Part model, mm, in its own coordinate system. A direction names the side the tool comes from. Round coordinates to 2 decimals unless told otherwise and drop trailing zeros.
(1) Cut at A-A on y = -2.5. Count the separate pieces of the cut face and the enclosed holes in it, then the cut area to 3 significant figures.
(2) Tool access for faces 1 (the face through (2, -6.5, 2)), 2 (the face through (-17, -3.5, 1)): list every direction of +Z, -Z, +X, -X, +Y, -Y with a clear straight run to the whole face (end or side of a thin tool).
(3) Mould opens along Z. For faces 3 (the face through (-77, -3.5, 1)), 4 (the face through (2, -3, -4.5)), 5 (the face through (-150, -3, 0)) say: +Z half, -Z half, draft (parallel to the pull), parting line (faces both ways), or undercut.
(4) Flat gauge pins, fed straight in: pin 1 (3 mm diameter, centred on x = -120, z = -0.5, fed in from +Y); pin 2 (1.8 mm diameter, centred on x = 81.5, z = 0, fed in from -Y); pin 3 (3.5 mm diameter, centred on x = -138.5, z = 0, fed in from +Y). Where does each tip first touch, or does it go through?
(5) Probe probe 1 along Z at (x, y) = (141.5, -2.3); probe 2 along Z at (x, y) = (-78.5, -4.7); probe 3 along Y at (x, z) = (120, -2). List the from-to ranges inside material, lowest first.
from build123d import *

# Parameters (mm, degrees)
SKETCH1_W           = 9
SKETCH1_H           = 6.5
BOSS_EXTRUDE1_DEPTH = 150
SKETCH2_R           = 1.5
CUT_EXTRUDE1_DEPTH  = 151.208188858
SKETCH3_R           = 3
CUT_EXTRUDE2_DEPTH  = 3.5


with BuildPart() as part:
    # Sketch1 → Boss-Extrude1 (new, symmetric)
    with BuildSketch(Plane(origin=(0, 0, 0), x_dir=(0, 0, -1), z_dir=(1, 0, 0))):
        with Locations((0, -3.25)):
            Rectangle(SKETCH1_W, SKETCH1_H)
    extrude(amount=BOSS_EXTRUDE1_DEPTH, both=True)

    # Sketch2 → Cut-Extrude1 (cut, through all)
    with BuildSketch(Plane(origin=(0, 0, 0), x_dir=(1, 0, 0), z_dir=(0, 1, 0))):
        with Locations(Location((-138.5, 0, 0), (0, 0, 270))):
            Circle(SKETCH2_R)
        with Locations(Location((-118.5, 0, 0), (0, 0, 270))):
            Circle(SKETCH2_R)
        with Locations(Location((-98.5, 0, 0), (0, 0, 270))):
            Circle(SKETCH2_R)
        with Locations(Location((-78.5, 0, 0), (0, 0, 270))):
            Circle(SKETCH2_R)
        with Locations(Location((-58.5, 0, 0), (0, 0, 270))):
            Circle(SKETCH2_R)
        with Locations(Location((-38.5, 0, 0), (0, 0, 270))):
            Circle(SKETCH2_R)
        with Locations(Location((-18.5, 0, 0), (0, 0, 270))):
            Circle(SKETCH2_R)
        with Locations(Location((1.5, 0, 0), (0, 0, 270))):
            Circle(SKETCH2_R)
        with Locations(Location((21.5, 0, 0), (0, 0, 270))):
            Circle(SKETCH2_R)
        with Locations(Location((41.5, 0, 0), (0, 0, 270))):
            Circle(SKETCH2_R)
        with Locations(Location((61.5, 0, 0), (0, 0, 270))):
            Circle(SKETCH2_R)
        with Locations(Location((81.5, 0, 0), (0, 0, 270))):
            Circle(SKETCH2_R)
        with Locations(Location((101.5, 0, 0), (0, 0, 270))):
            Circle(SKETCH2_R)
        with Locations(Location((121.5, 0, 0), (0, 0, 270))):
            Circle(SKETCH2_R)
        with Locations(Location((141.5, 0, 0), (0, 0, 270))):
            Circle(SKETCH2_R)
    extrude(amount=-CUT_EXTRUDE1_DEPTH, mode=Mode.SUBTRACT)

    # Sketch3 → Cut-Extrude2 (cut)
    with BuildSketch(Plane(origin=(0, 0, 0), x_dir=(1, 0, 0), z_dir=(0, 1, 0))):
        with Locations(Location((-138.5, 0, 0), (0, 0, 270))):
            Circle(SKETCH3_R)
        with Locations(Location((-118.5, 0, 0), (0, 0, 270))):
            Circle(SKETCH3_R)
        with Locations(Location((-98.5, 0, 0), (0, 0, 270))):
            Circle(SKETCH3_R)
        with Locations(Location((-78.5, 0, 0), (0, 0, 270))):
            Circle(SKETCH3_R)
        with Locations(Location((-58.5, 0, 0), (0, 0, 270))):
            Circle(SKETCH3_R)
        with Locations(Location((-38.5, 0, 0), (0, 0, 270))):
            Circle(SKETCH3_R)
        with Locations(Location((-18.5, 0, 0), (0, 0, 270))):
            Circle(SKETCH3_R)
        with Locations(Location((1.5, 0, 0), (0, 0, 270))):
            Circle(SKETCH3_R)
        with Locations(Location((21.5, 0, 0), (0, 0, 270))):
            Circle(SKETCH3_R)
        with Locations(Location((41.5, 0, 0), (0, 0, 270))):
            Circle(SKETCH3_R)
        with Locations(Location((61.5, 0, 0), (0, 0, 270))):
            Circle(SKETCH3_R)
        with Locations(Location((81.5, 0, 0), (0, 0, 270))):
            Circle(SKETCH3_R)
        with Locations(Location((101.5, 0, 0), (0, 0, 270))):
            Circle(SKETCH3_R)
        with Locations(Location((121.5, 0, 0), (0, 0, 270))):
            Circle(SKETCH3_R)
        with Locations(Location((141.5, 0, 0), (0, 0, 270))):
            Circle(SKETCH3_R)
    extrude(amount=-CUT_EXTRUDE2_DEPTH, mode=Mode.SUBTRACT)


solid = part.part
Final values:
1. separate pieces: 1
1. enclosed holes: 15
1. area: 2,280 mm2
2. face 1: +Z, -Z, +X, -X, -Y
2. face 2: +Y
3. face 3: undercut
3. face 4: -Z half
3. face 5: draft
4. pin 1: stops at y = 0
4. pin 2: passes through
4. pin 3: stops at y = -3.5
5. probe 1: z = -4.5 to -3, 3 to 4.5
5. probe 2: z = -4.5 to -1.5, 1.5 to 4.5
5. probe 3: y = -6.5 to -3.5
